```python
from build123d import *

# Parameters (mm, degrees)
ESQUISSE1_W             = 200
ESQUISSE1_H             = 100
BOSS_EXTRU_1_DEPTH      = 100
CHANFREIN1_SIZE         = 40
ESQUISSE2_R             = 6.5
ENL_V_MAT_EXTRU_1_DEPTH = 230.128784748
ESQUISSE4_R             = 1.5
ENL_V_MAT_EXTRU_3_DEPTH = 151
ESQUISSE5_W             = 144
ESQUISSE5_H             = 84
ENL_V_MAT_EXTRU_4_DEPTH = 75
ESQUISSE6_W             = 152
ESQUISSE6_H             = 92
ENL_V_MAT_EXTRU_5_DEPTH = 8


with BuildPart() as part:
    # Esquisse1 → Boss.-Extru.1 (new body)
    with BuildSketch(Plane.XY):
        Rectangle(ESQUISSE1_W, ESQUISSE1_H)
    extrude(amount=BOSS_EXTRU_1_DEPTH)

    # Chanfrein1
    chanfrein1_edges = [part.edges().sort_by_distance(p)[0] for p in [
        (-100, -50, 50),
    ]]
    chamfer(chanfrein1_edges, length=CHANFREIN1_SIZE)

    # Esquisse2 → Enlèv. mat.-Extru.1 (cut, through all)
    with BuildSketch(Plane(origin=(100, 0, 0), x_dir=(0, 0, -1), z_dir=(1, 0, 0))):
        with Locations((-50, 30)):
            Circle(ESQUISSE2_R)
    extrude(amount=-ENL_V_MAT_EXTRU_1_DEPTH, mode=Mode.SUBTRACT)

    # Esquisse4 → Enlèv. mat.-Extru.3 (cut, through all)
    with BuildSketch(Plane.XY.offset(100)):
        with Locations((85, -45)):
            Circle(ESQUISSE4_R)
        with Locations((-40, -45)):
            Circle(ESQUISSE4_R)
    extrude(amount=-ENL_V_MAT_EXTRU_3_DEPTH, mode=Mode.SUBTRACT)

    # Esquisse5 → Enlèv. mat.-Extru.4 (cut)
    with BuildSketch(Plane.XZ.offset(50)):
        with Locations((20, 50)):
            Rectangle(ESQUISSE5_W, ESQUISSE5_H)
    extrude(amount=-ENL_V_MAT_EXTRU_4_DEPTH, mode=Mode.SUBTRACT)

    # Esquisse6 → Enlèv. mat.-Extru.5 (cut)
    with BuildSketch(Plane.XZ.offset(50)):
        with Locations((20, 50)):
            Rectangle(ESQUISSE6_W, ESQUISSE6_H)
    extrude(amount=-ENL_V_MAT_EXTRU_5_DEPTH, mode=Mode.SUBTRACT)


solid = part.part
```
The listing builds one solid part. Answer for the finished solid, in the listing's coordinates (mm). A direction names the side the tool comes from. Round coordinates to 2 decimals unless told otherwise and drop trailing zeros. Loops run counter-clockwise (first coordinate to the right, second up) from the corner with the lowest first, then second, coordinate; pieces in that order, holes last.
Q1. Section D-D, the plane y = 5 is taken. Determine the outline of the cut face in (x, z).
Q2. Section C-C, the plane x = -85 is taken. Determine the outline of the cut face in (y, z), then the cut area to 3 significant figures.
Q3. Which of the six approach directions +Z, -Z, +X, -X, +Y, -Y give full straight-line access (tool end or side, diameter ignored) to faces 4 (the face through (19, -9, 92)), 5 (the face through (1.4, 36.445, 50.846))?
Q4. Section A-A, the plane y = 30 is taken. Determine the outline of the cut face in (x, z).
Q5. Find the intervals of material crossed by line 1 (X direction, y = 4, z = 91); line 2 (Z direction, x = 81, y = 23); line 3 (Y direction, x = 85, z = 98.1), in increasing order.
Q6. Given pin 1 Ø4 at (x, z) = (71, 54.5) entering from -Y; pin 2 Ø9 at (x, y) = (48.5, -46) entering from -Z; pin 3 Ø2.5 at (x, y) = (85, -45) entering from -Z; pin 4 Ø12 at (y, z) = (-23, 78) entering from -X, each flat-ended and moving along its own axis, determine where each tip first touches the part or whether it passes through.
Q7. Section B-B, the plane z = 50 is taken. Determine the outline of the cut face in (x, y).
Q8. For a pull along Z with two mould halves and no side action, classify faces 1 (the face through (19, -9, 8)), 2 (the face through (-1, 1, 0)), 3 (the face through (14, -50, 98)) as released by +Z, released by -Z, zero draft, split by the parting line, or undercut.
Completed:
1. outline: (-100, 0) - (100, 0) - (100, 100) - (-100, 100) - close; hole (-52, 8) - (92, 8) - (92, 92) - (-52, 92) - close
2. outline: (-25, 0) - (50, 0) - (50, 100) - (-25, 100) - close; hole circle Ø13 at (30, 50)
2. area: 7,370 mm2
3. face 4: -Y
3. face 5: +X, -X
4. outline: (-100, 0) - (100, 0) - (100, 43.5) - (-100, 43.5) - close; (-100, 56.5) - (100, 56.5) - (100, 100) - (-100, 100) - close
5. line 1: x = -100 to -52, 92 to 100
5. line 2: z = 0 to 8, 92 to 100
5. line 3: y = -50 to -46.5, -43.5 to 50
6. pin 1: stops at y = 25
6. pin 2: stops at z = 0
6. pin 3: passes through
6. pin 4: stops at x = -93
7. outline: (-100, -10) - (-60, -50) - (-56, -50) - (-56, -42) - (-52, -42) - (-52, 23.5) - (-100, 23.5) - close; (-100, 36.5) - (100, 36.5) - (100, 50) - (-100, 50) - close; (92, -42) - (96, -42) - (96, -50) - (100, -50) - (100, 23.5) - (92, 23.5) - close
8. face 1: undercut
8. face 2: released by -Z
8. face 3: zero draft
